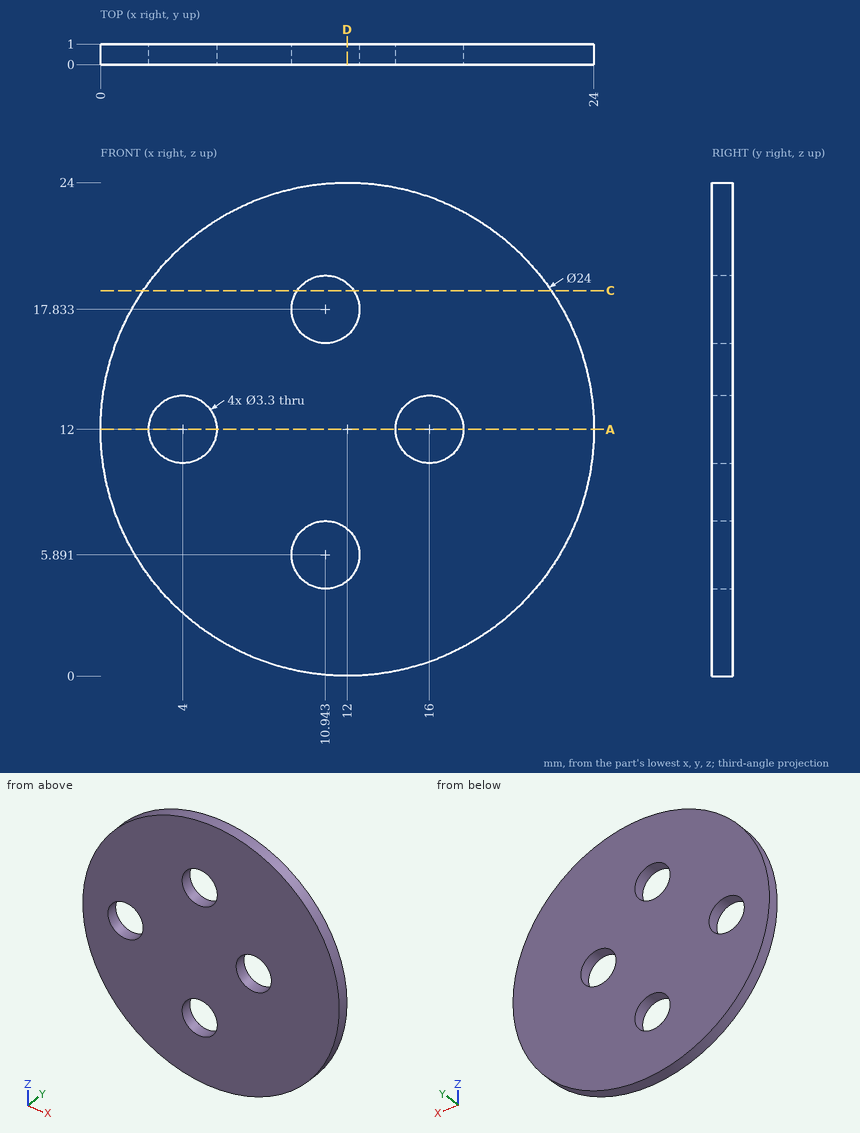
Source: three-view drawing plus pictorial views. Frame: mm from the lowest corner of the part. Give positions to 0.01 mm unless a question says otherwise; leave off trailing zeros. Loops run counter-clockwise (first coordinate to the right, second up) from the corner with the lowest first, then second, coordinate; pieces in that order, holes last.
1) Line query: L1, parallel to X at y = 0.2, z = 10.5 (1 decimal); L2, parallel to Z at x = 11, y = 0.65; L3, parallel to Z at x = 10, y = 0.5 (1 decimal). Output: solid intervals per line, ascending.
A:
L1: x = 0.1 to 3.3, 4.7 to 15.3, 16.7 to 23.9
L2: z = 0.04 to 4.24, 7.54 to 16.18, 19.48 to 23.96
L3: z = 0.2 to 4.5, 7.2 to 16.5, 19.2 to 23.8
2) Section query A-A on z = 12. Return the cut outline in (x, y), and give its area (3 significant figures).
A:
outline: (0, 0) - (2.35, 0) - (2.35, 1) - (0, 1) - close; (5.65, 0) - (14.35, 0) - (14.35, 1) - (5.65, 1) - close; (17.65, 0) - (24, 0) - (24, 1) - (17.65, 1) - close
area: 17.4 mm2
3) Section query D-D on x = 12. Return the cut outline in (y, z) (1 decimal).
A:
outline: (0, 0) - (1, 0) - (1, 4.6) - (0, 4.6) - close; (0, 7.2) - (1, 7.2) - (1, 16.6) - (0, 16.6) - close; (0, 19.1) - (1, 19.1) - (1, 24) - (0, 24) - close
4) Section query C-C on z = 18.75. Return the cut outline in (x, y) (1 decimal), and give its area (3 significant figures).
A:
outline: (2.1, 0) - (9.6, 0) - (9.6, 1) - (2.1, 1) - close; (12.3, 0) - (21.9, 0) - (21.9, 1) - (12.3, 1) - close
area: 17.1 mm2
